Build history of the part. All positions in model axes, mm. Face numbers are marked on the shaded views. A direction names the side the tool comes from. Coordinates: 2 decimals unless noted, no trailing zeros. Write each loop counter-clockwise with the first axis right and the second up, starting at its lowest first coordinate (ties: lowest second). Pieces come first, ordered by that corner, then holes. Notation, with made-up numbers: M 88.5,77 L 114.5,77 A19 cw 114.5,111 Z; hole C -4.5,22.25 d2. An arc over 180 degrees is marked long. Use CSV: the item, a comma, the result in double quotes. Start each with the question number.
```python
from build123d import *

# Parameters (mm, degrees)
F0_W     = 50.8
F0_H     = 50.8
F2_DEPTH = 25.4
F1_R     = 14.28115
F3_DEPTH = 7.9375
F4_R     = 14.28115
F5_DEPTH = 7.9375
F6_R     = 11.1125
F7_DEPTH = 25.4


with BuildPart() as f2:
    # F0 (on Front) → F2 (new body)
    with BuildSketch(Plane.XZ):
        with Locations((-25.4, 32.4630600569)):
            Rectangle(F0_W, F0_H)
    extrude(amount=F2_DEPTH)

    # F1 (on Front) → F3 (cut)
    with BuildSketch(Plane.XZ):
        with Locations((-25.4, 32.4630600569)):
            Circle(F1_R)
    extrude(amount=F3_DEPTH, mode=Mode.SUBTRACT)

    # F4 (on face) → F5 (cut)
    with BuildSketch(Plane.XZ.offset(25.4)):
        with Locations((-25.4, 32.4630600569)):
            Circle(F4_R)
    extrude(amount=-F5_DEPTH, mode=Mode.SUBTRACT)

    # F6 (on face) → F7 (cut)
    with BuildSketch(Plane.XZ.offset(17.4625)):
        with Locations((-25.4, 32.4630600569)):
            Circle(F6_R)
    extrude(amount=-F7_DEPTH, mode=Mode.SUBTRACT)


solid = f2.part
```
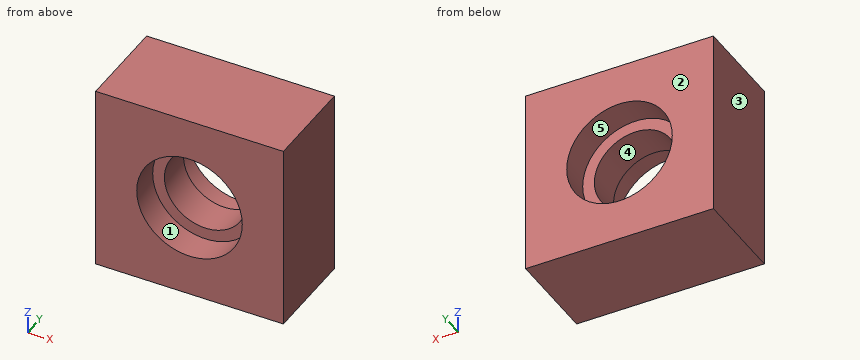
1. Slice it at A-A (x = -25.4). List the corners of the cut face in (y, z).
2. Slice it at B-B (z = 31.5). List the corners of the cut face in (x, y), and give its area (3 significant figures).
3. 3-axis set-ups, long thin cutter, end or side, ignore diameter. For the marked faces 4 and 5: which of +Z, -Z, +X, -X, +Y, -Y reach the whole face in a straight line?
4. Slice it at D-D (y = -16.5). List the corners of the cut face in (x, z) (1 decimal), and give its area (3 significant figures).
5. Slice it at C-C (y = -4). List the corners of the cut face in (x, z).
6. Drill centre lines: line 1 along X through (y, z) = (-20.75, 32); line 2 along Z through (x, y) = (-25.4, -3.75); line 3 along Y through (x, z) = (-12, 30.5). Where is each one in solid material? Low to high. Write a range as from..to.
7. Pull direction X, two halves, no side cores. Call the marked faces 1, 2 and 3: pulls with the +X half, pulls with the -X half, needs draft (parallel to the pull), parting line crosses it, or undercut.
Established:
1,outline,"M -25.4,7.06 L 0,7.06 L 0,18.18 L -7.94,18.18 L -7.94,21.35 L -17.46,21.35 L -17.46,18.18 L -25.4,18.18 Z; M -25.4,46.74 L -17.46,46.74 L -17.46,43.58 L -7.94,43.58 L -7.94,46.74 L 0,46.74 L 0,57.86 L -25.4,57.86 Z"
2,outline,"M -50.8,-25.4 L -39.65,-25.4 L -39.65,-17.46 L -36.47,-17.46 L -36.47,-7.94 L -39.65,-7.94 L -39.65,0 L -50.8,0 Z; M -14.33,-17.46 L -11.15,-17.46 L -11.15,-25.4 L 0,-25.4 L 0,0 L -11.15,0 L -11.15,-7.94 L -14.33,-7.94 Z"
2,area,"627 mm2"
3,face 4,"+Y, -Y"
3,face 5,"+Y"
4,outline,"M -50.8,7.1 L 0,7.1 L 0,57.9 L -50.8,57.9 Z; hole C -25.4,32.5 d22.2"
4,area,"2,190 mm2"
5,outline,"M -50.8,7.06 L 0,7.06 L 0,57.86 L -50.8,57.86 Z; hole C -25.4,32.46 d28.56"
6,line 1,"x = -50.8..-39.67, -11.13..0"
6,line 2,"z = 7.06..18.18, 46.74..57.86"
6,line 3,"y = -17.46..-7.94"
7,face 1,"undercut"
7,face 2,"needs draft"
7,face 3,"pulls with the -X half"
